Autodesk Inventor part; units mm, degrees
ref_plane "YZ Plane" through (0, 0, 0) normal (1, 0, 0) x (0, 1, 0)
ref_plane "XZ Plane" through (0, 0, 0) normal (0, 1, 0) x (-1, 0, 0)
ref_plane "XY Plane" through (0, 0, 0) normal (0, 0, 1) x (1, 0, 0)
sketch "Sketch1" plane through (0, 0, 0) normal (0, 0, 1) x (1, 0, 0)
  line L0 (0, 0) -> (33, 0)
  line L1 (33, 0) -> (33, 28)
  line L2 (33, 28) -> (0, 28)
  line L3 (0, 28) -> (0, 0)
  circle A0 centre (16.5, 14) radius 4
  circle A1 centre (16.5, 23.5) radius 1.5
  circle A2 centre (9, 5) radius 1.5
  circle A3 centre (24, 5) radius 1.5
  dimension "d0" = 33
  dimension "d1" = 28
  dimension "d2" = 8
  dimension "d3" = 14
  dimension "d4" = 16.5
  dimension "d5" = 3
  dimension "d6" = 3
  dimension "d7" = 3
  dimension "d8" = 4.5
  dimension "d9" = 0
  dimension "d10" = 15
  dimension "d11" = 5
  dimension "d12" = 9
  dimension "d13" = 5
extrude "Extrusion1" add sketch "Sketch1" along normal blind 3
sketch "Sketch2" plane through (0, 0, 3) normal (0, 0, 1) x (1, 0, 0)
  circle A0 centre (16.5, 14) radius 4
  circle A1 centre (16.5, 14) radius 5.425
  point P0 (0, 0)
  dimension "d16" = 10.85
extrude "Extrusion2" cut sketch "Sketch2" against normal blind 2 contours A0 | A1
fillet "Fillet1" radius 15 2 edges at (33, 28, 1.5) (0, 28, 1.5)
sketch "Sketch3" plane through (0, 0, 3) normal (0, 0, 1) x (1, 0, 0)
  arc A0 (15, 28) -> (0, 13) centre (15, 13) ccw
  line L0 (0, 13) -> (0, 0)
  line L1 (0, 0) -> (33, 0)
  line L2 (33, 0) -> (33, 13)
  arc A1 (33, 13) -> (18, 28) centre (18, 13) ccw
  line L3 (18, 28) -> (15, 28)
  circle A2 centre (16.5, 14) radius 5.425
  circle A3 centre (16.5, 23.5) radius 1.5
  circle A4 centre (9, 5) radius 1.5
  circle A5 centre (24, 5) radius 1.5
equation "\"d3\" = 0.5 * d1"
equation "\"d4\" = 0.5 * d0"
properties part number "Arm6_3D" material "Aluminum 6061, Welded"
Geometry: final body of the model. Coordinates: model frame, mm. A direction names the side the tool comes from. Round coordinates to 2 decimals unless told otherwise and drop trailing zeros. Write each loop counter-clockwise with the first axis right and the second up, starting at its lowest first coordinate (ties: lowest second). Pieces come first, ordered by that corner, then holes.
Item 1: Section query D-D (y = 14). Return loops of the section in (x, z) (3 decimals).
Item 2: Section query B-B (z = 1.8). Return loops of the section in (x, y) (3 decimals).
Item 3: Section query C-C (y = 5). Return loops of the section in (x, z).
Item 4: Section query A-A (x = 16.5). Return loops of the section in (y, z) (3 decimals), plus the area to 3 significant figures.
Item 5: Pin query (flat end, axial travel): P1, Ø1.5, axis at x = 27, z = 0.5, coming from the +Y side; P2, Ø5.5, axis at x = 15, y = 14, coming from the +Z side. Return the tip coordinate at first contact, or that it passes through.
Item 6: Mould query, pull axis X, two halves, no side actions, for faces 1 (the face through (28.72, 23.49, 1.52)), 2 (the face through (7.89, 3.99, 1.48)), 3 (the face through (17, 28, 1)). Classes: +X half, -X half, draft (parallel to the pull), parting line (faces both ways), or undercut.
Item 7: Material intervals for L1, parallel to Y at x = 16.5, z = 0.5; L2, parallel to Y at x = 16.5, z = 2.3 (3 decimals); L3, parallel to Y at x = 6, z = 2.5, sorted ascending.
Item 8: Set-up query: faces 4 (the face through (0, 7, 1)), 5 (the face through (19.003, 9.187, 2.014)). Return all of +Z, -Z, +X, -X, +Y, -Y with unobstructed straight access to the full face (end or side cutting, diameter ignored); none if empty.
Completed:
1. outline: (0.033, 0) - (12.5, 0) - (12.5, 1) - (11.075, 1) - (11.075, 3) - (0.033, 3) - close; (20.5, 0) - (32.967, 0) - (32.967, 3) - (21.925, 3) - (21.925, 1) - (20.5, 1) - close
2. outline: (0, 0) - (33, 0) - (33, 13) arc R15 ccw to (18, 28) - (15, 28) arc R15 ccw to (0, 13) - close; hole circle Ø3 at (9, 5); hole circle Ø10.85 at (16.5, 14); hole circle Ø3 at (16.5, 23.5); hole circle Ø3 at (24, 5)
3. outline: (0, 0) - (7.5, 0) - (7.5, 3) - (0, 3) - close; (10.5, 0) - (22.5, 0) - (22.5, 3) - (10.5, 3) - close; (25.5, 0) - (33, 0) - (33, 3) - (25.5, 3) - close
4. outline: (0, 0) - (10, 0) - (10, 1) - (8.575, 1) - (8.575, 3) - (0, 3) - close; (18, 0) - (22, 0) - (22, 3) - (19.425, 3) - (19.425, 1) - (18, 1) - close; (25, 0) - (28, 0) - (28, 3) - (25, 3) - close
4. area: 45.3 mm2
5. P1: stops at y = 25.53
5. P2: stops at z = 1
6. face 1: +X half
6. face 2: undercut
6. face 3: draft
7. L1: y = 0 to 10, 18 to 22, 25 to 28
7. L2: y = 0 to 8.575, 19.425 to 22, 25 to 28
7. L3: y = 0 to 25
8. face 4: +Z, -Z, -X, +Y, -Y
8. face 5: +Z
